from build123d import *

# Parameters (mm, degrees)
ESQUISSE1_W             = 150
ESQUISSE1_H             = 70
BOSS_EXTRU_1_DEPTH      = 25
ESQUISSE2_W             = 66
ESQUISSE2_H             = 58
ENL_V_MAT_EXTRU_1_DEPTH = 15
ESQUISSE3_R             = 25
ESQUISSE3_R_2           = 20
BOSS_EXTRU_2_DEPTH      = 5
ESQUISSE4_R             = 25
ESQUISSE4_R_2           = 20
ENL_V_MAT_EXTRU_2_DEPTH = 5
ESQUISSE5_R             = 7.5
BOSS_EXTRU_3_DEPTH      = 10
CONG_2_R                = 3
ESQUISSE6_R             = 2.5
BOSS_EXTRU_4_DEPTH      = 5
ESQUISSE7_R             = 4.575268676
BOSS_EXTRU_5_DEPTH      = 10


with BuildPart() as part:
    # Esquisse1 → Boss.-Extru.1 (new body)
    with BuildSketch(Plane.XY):
        with Locations((75, 35)):
            Rectangle(ESQUISSE1_W, ESQUISSE1_H)
    extrude(amount=BOSS_EXTRU_1_DEPTH)

    # Esquisse2 → Enlèv. mat.-Extru.1 (cut)
    with BuildSketch(Plane.XY.offset(25)):
        with Locations((39, 35)):
            Rectangle(ESQUISSE2_W, ESQUISSE2_H)
        with Locations((111, 35)):
            Rectangle(ESQUISSE2_W, ESQUISSE2_H)
    extrude(amount=-ENL_V_MAT_EXTRU_1_DEPTH, mode=Mode.SUBTRACT)

    # Esquisse3 → Boss.-Extru.2 (add)
    with BuildSketch(Plane.XY.offset(10)):
        with Locations((37.5, 35)):
            Circle(ESQUISSE3_R)
        with Locations((37.5, 35)):
            Circle(ESQUISSE3_R_2, mode=Mode.SUBTRACT)
    extrude(amount=BOSS_EXTRU_2_DEPTH)

    # Esquisse4 → Enlèv. mat.-Extru.2 (cut)
    with BuildSketch(Plane.XY.offset(10)):
        with Locations((112.5, 35)):
            Circle(ESQUISSE4_R)
        with Locations((112.5, 35)):
            Circle(ESQUISSE4_R_2, mode=Mode.SUBTRACT)
    extrude(amount=-ENL_V_MAT_EXTRU_2_DEPTH, mode=Mode.SUBTRACT)

    # Esquisse5 → Boss.-Extru.3 (add)
    with BuildSketch(Plane.XY.offset(10)):
        with Locations((37.5, 35)):
            Circle(ESQUISSE5_R)
    extrude(amount=BOSS_EXTRU_3_DEPTH)

    # Congé2
    cong_2_edges = [part.edges().sort_by_distance(p)[0] for p in [
        (30, 35, 20),
    ]]
    fillet(cong_2_edges, radius=CONG_2_R)

    # Esquisse6 → Boss.-Extru.4 (add)
    with BuildSketch(Plane.XY.offset(10)):
        with Locations((112.5, 35)):
            Circle(ESQUISSE6_R)
    extrude(amount=BOSS_EXTRU_4_DEPTH)

    # Esquisse7 → Boss.-Extru.5 (add)
    with BuildSketch(Plane.XY.offset(20)):
        with Locations((37.5, 35)):
            Circle(ESQUISSE7_R)
    extrude(amount=BOSS_EXTRU_5_DEPTH)


solid = part.part
Check sheet for the modelled part. Datum: model origin and axes. Units: mm. A direction names the side the tool comes from. Give positions to 0.01 mm unless a question says otherwise; leave off trailing zeros. Write each loop counter-clockwise with the first axis right and the second up, starting at its lowest first coordinate (ties: lowest second). Pieces come first, ordered by that corner, then holes. Notation, with made-up numbers: (51.5, 4) -> (99.5, 4) arc R17 ccw to (99.5, 11) -> close; hole circle Ø2 at (76, 62.25). An arc over 180 degrees is marked (long way). One line per item, written item: value. Start each with the question number.
Item 1: Draft check along X on faces 1 (the flat face through (101, 52, 5)), 2 (the flat face through (74, 70, 12)), 3 (the flat face through (0, 35, 12)). Enter one of: +X half, -X half, draft (parallel to the pull), parting line (faces both ways), or undercut.
Item 2: Material ranges on probe 1 along X at (y, z) = (61, 22.75); probe 2 along Y at (x, z) = (112.5, 7.15); probe 3 along Y at (x, z) = (37.5, 13.3), recorded low to high. Write a range as from..to.
Item 3: Gauge pin test, flat ends, axial feed: pin 1 (17.5 mm diameter, centred on x = 23, y = 44, fed in from +Z); pin 2 (12 mm diameter, centred on x = 30, y = 45, fed in from +Z); pin 3 (10 mm diameter, centred on x = 84.5, y = 59.5, fed in from +Z). Record the tip position at first contact, or that the pin passes through.
Item 4: Tool access check on faces 4 (the flat face through (37, 35, 30)), 5 (the flat face through (26, 52, 15)). Record the directions out of +Z, -Z, +X, -X, +Y, -Y that give a thin tool (end or side, any length) a straight path to the whole face; none if there is none.
Item 5: Section check A-A on z = 12. Record the cut outline in (x, y).
Item 6: Section check C-C on x = 37.5. Record the cut outline in (y, z), then the cut area to 3 significant figures.
Item 7: Section check D-D on y = 13.5. Record the cut outline in (x, z), then the cut area to 3 significant figures.
Item 8: Section check B-B on x = 139.5. Record the cut outline in (y, z), then the cut area to 3 significant figures.
Results list:
1. face 1: undercut
1. face 2: draft
1. face 3: -X half
2. probe 1: 0..6, 72..78, 144..150
2. probe 2: 0..10, 15..55, 60..70
2. probe 3: 0..6, 10..15, 27.5..42.5, 55..60, 64..70
3. pin 1: z = 15
3. pin 2: z = 19.24
3. pin 3: z = 25
4. face 4: +Z, +X, -X, +Y, -Y
4. face 5: +Z
5. outline: (0, 0) -> (150, 0) -> (150, 70) -> (0, 70) -> close; circle Ø50 at (37.5, 35); circle Ø15 at (37.5, 35); circle Ø5 at (112.5, 35); hole (6, 6) -> (72, 6) -> (72, 64) -> (6, 64) -> close; hole circle Ø40 at (37.5, 35); hole (78, 6) -> (144, 6) -> (144, 64) -> (78, 64) -> close
6. outline: (0, 0) -> (70, 0) -> (70, 25) -> (64, 25) -> (64, 10) -> (60, 10) -> (60, 15) -> (55, 15) -> (55, 10) -> (42.5, 10) -> (42.5, 17) arc R3 ccw to (39.5, 20) -> (39.58, 20) -> (39.58, 30) -> (30.42, 30) -> (30.42, 20) -> (30.5, 20) arc R3 ccw to (27.5, 17) -> (27.5, 10) -> (15, 10) -> (15, 15) -> (10, 15) -> (10, 10) -> (6, 10) -> (6, 25) -> (0, 25) -> close
6. area: 1,170 mm²
7. outline: (0, 0) -> (150, 0) -> (150, 25) -> (144, 25) -> (144, 10) -> (125.26, 10) -> (125.26, 5) -> (99.74, 5) -> (99.74, 10) -> (78, 10) -> (78, 25) -> (72, 25) -> (72, 10) -> (50.26, 10) -> (50.26, 15) -> (24.74, 15) -> (24.74, 10) -> (6, 10) -> (6, 25) -> (0, 25) -> close
7. area: 1,770 mm²
8. outline: (0, 0) -> (70, 0) -> (70, 25) -> (64, 25) -> (64, 10) -> (6, 10) -> (6, 25) -> (0, 25) -> close
8. area: 880 mm²
